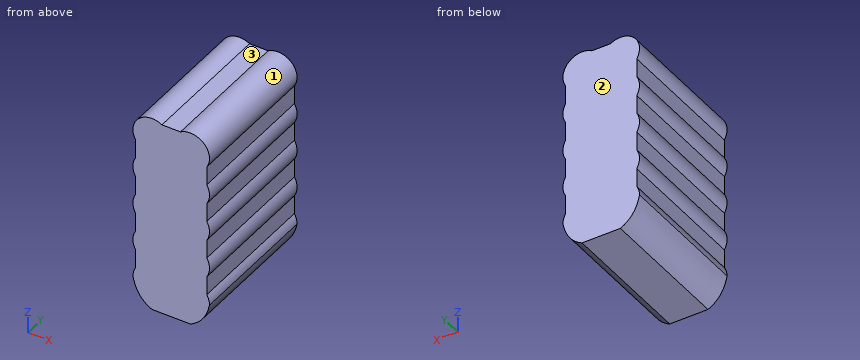
```python
from build123d import *

# Parameters (mm, degrees)
BOSS_EXTRUDE1_DEPTH = 50


with BuildPart() as part:
    # Sketch2 → Boss-Extrude1 (new body)
    with BuildSketch(Plane(origin=(0, 0, 0), x_dir=(1, 0, 0), z_dir=(0, 1, 0))):
        with BuildLine():
            Line((7, 38), (-7, 38))
            add(Edge.make_bspline(
                [(-7, 38), (-12.596418812, 35.328912619), (-14, 28)],
                knots=[0.092966826, 0.092966826, 0.092966826, 0.41073738, 0.41073738, 0.41073738], degree=2))
            ThreePointArc((-14, 28), (-13.745368782, 26.129171307), (-13, 24.394448725))
            Line((-13, 24.394448725), (-13, 17.605551275))
            ThreePointArc((-13, 17.605551275), (-14, 14), (-13, 10.394448725))
            Line((-13, 10.394448725), (-13, 3.605551275))
            ThreePointArc((-13, 3.605551275), (-14, 0), (-13, -3.605551275))
            Line((-13, -3.605551275), (-13, -10.394448725))
            ThreePointArc((-13, -10.394448725), (-14, -14), (-13, -17.605551275))
            Line((-13, -17.605551275), (-13, -24.394448725))
            ThreePointArc((-13, -24.394448725), (-11.949747468, -32.949747468), (-3.394448725, -34))
            Line((-3.394448725, -34), (3.394448725, -34))
            ThreePointArc((3.394448725, -34), (11.949747468, -32.949747468), (13, -24.394448725))
            Line((13, -24.394448725), (13, -17.605551275))
            ThreePointArc((13, -17.605551275), (14, -14), (13, -10.394448725))
            Line((13, -10.394448725), (13, -3.605551275))
            ThreePointArc((13, -3.605551275), (14, 0), (13, 3.605551275))
            Line((13, 3.605551275), (13, 10.394448725))
            ThreePointArc((13, 10.394448725), (14, 14), (13, 17.605551275))
            Line((13, 17.605551275), (13, 24.394448725))
            ThreePointArc((13, 24.394448725), (13.745368782, 26.129171307), (14, 28))
            add(Edge.make_bspline(
                [(14, 28), (12.596418812, 35.328912619), (7, 38)],
                knots=[0.907033174, 0.907033174, 0.907033174, 1.224803727, 1.224803727, 1.224803727], degree=2))
        make_face()
    extrude(amount=BOSS_EXTRUDE1_DEPTH)


solid = part.part
```
CAD build for the part. Positions are in the model's coordinates, mm. Face numbers are marked on the shaded views. Round coordinates to 2 decimals unless told otherwise and drop trailing zeros. Order: outer loops, then holes, each group sorted by start corner. A loop starts at its lowest first (then second) coordinate and runs counter-clockwise, first axis right, second up.
Q1. Slice it at A-A (z = -23). Write the cut outline in (x, y), and give its area (3 significant figures).
Q2. Two-plate mould, pull along X, no slides. Class the marked faces 1, 2 and 3: pulls with the +X half, pulls with the -X half, needs draft (parallel to the pull), parting line crosses it, or undercut.
Q3. Wall check: L1, parallel to X at y = 6, z = 8.5; L2, parallel to Z at x = -0.5, y = 10; L3, parallel to X at y = 39, z = -0.5. Give the ranges that are in metal, low to high.
Q4. Drop flat-ended pins along their axis: pin 1 (5.5 mm diameter, centred on y = 31.5, z = 6.5, fed in from -X); pin 2 (2 mm diameter, centred on y = 31.5, z = -20, fed in from +X); pin 3 (2 mm diameter, centred on x = -1, y = 34.5, fed in from +Z). Give the stop position or say it passes through.
Results below:
1. outline: (-13, 0) - (13, 0) - (13, 50) - (-13, 50) - close
1. area: 1,300 mm2
2. face 1: undercut
2. face 2: needs draft
2. face 3: undercut
3. L1: x = -13 to 13
3. L2: z = -38 to 34
3. L3: x = -13.98 to 13.98
4. pin 1: stops at x = -13
4. pin 2: stops at x = 13
4. pin 3: stops at z = 34
